Read the model definition and answer for the solid it produces. Units are mm, in the model's axes. Face numbers are marked on the shaded views. A direction names the side the tool comes from. Give positions to 0.01 mm unless a question says otherwise; leave off trailing zeros. Order: outer loops, then holes, each group sorted by start corner. A loop starts at its lowest first (then second) coordinate and runs counter-clockwise, first axis right, second up. Notation, with made-up numbers: (14.25, 9) - (58.25, 9) arc R18 cw to (58.25, 25) - close; hole circle Ø8 at (40, 17.25). An arc over 180 degrees is marked (long way). Answer as CSV lines item,"result". Start each with the question number.
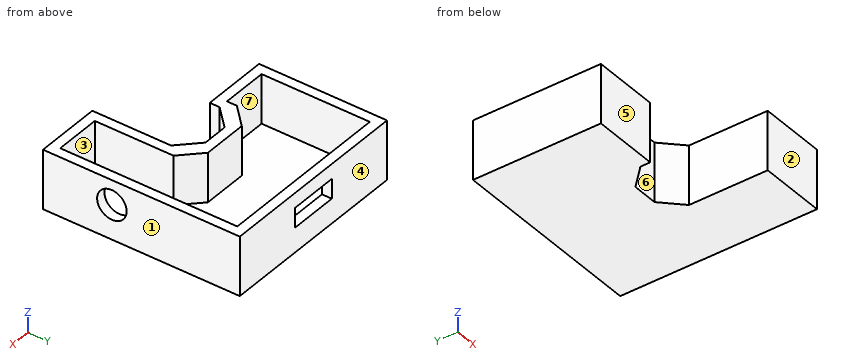
from build123d import *

# Parameters (mm, degrees)
BOSS_EXTRUDE1_DEPTH = 12.5
BOSS_EXTRUDE2_DEPTH = 5
SKETCH3_W           = 25
SKETCH3_H           = 10
CUT_EXTRUDE1_DEPTH  = 109.771549589
SKETCH4_R           = 7.5
CUT_EXTRUDE2_DEPTH  = 10
CHAMFER2_SIZE       = 10
CHAMFER3_SIZE       = 10


with BuildPart() as part:
    # Sketch1 → Boss-Extrude1 (new, symmetric)
    with BuildSketch(Plane.XY):
        Polygon((50, -50), (16.5, -50), (16.5, -45), (16.5, 0), (-16.5, 0), (-16.5, -15), (-50, -15), (-50, 50), (50, 50), align=None)
        Polygon((45, -45), (45, 45), (-45, 45), (-45, -10), (-21.5, -10), (-21.5, 5), (21.5, 5), (21.5, -45), align=None, mode=Mode.SUBTRACT)
    extrude(amount=BOSS_EXTRUDE1_DEPTH, both=True)

    # Sketch2 → Boss-Extrude2 (add)
    with BuildSketch(Plane(origin=(0, 0, -12.5), x_dir=(-1, 0, 0), z_dir=(0, 0, -1))):
        Polygon((-16.5, 0), (16.5, 0), (16.5, -15), (50, -15), (50, 50), (-50, 50), (-50, -50), (-16.5, -50), align=None)
    extrude(amount=BOSS_EXTRUDE2_DEPTH)

    # Sketch3 → Cut-Extrude1 (cut, through all)
    with BuildSketch(Plane.XZ.offset(-45)):
        Rectangle(SKETCH3_W, SKETCH3_H)
    extrude(amount=-CUT_EXTRUDE1_DEPTH, mode=Mode.SUBTRACT)

    # Sketch4 → Cut-Extrude2 (cut)
    with BuildSketch(Plane(origin=(50, 0, 0), x_dir=(0, 0, -1), z_dir=(1, 0, 0))):
        with Locations(Location((0, -15, 0), (0, 0, 90))):
            Circle(SKETCH4_R)
    extrude(amount=-CUT_EXTRUDE2_DEPTH, mode=Mode.SUBTRACT)

    # Chamfer2
    chamfer2_edges = [part.edges().sort_by_distance(p)[0] for p in [
        (16.5, 0, -2.5),
        (-16.5, 0, -2.5),
    ]]
    chamfer(chamfer2_edges, length=CHAMFER2_SIZE)

    # Chamfer3
    chamfer3_edges = [part.edges().sort_by_distance(p)[0] for p in [
        (-21.5, 5, 0),
        (21.5, 5, 0),
    ]]
    chamfer(chamfer3_edges, length=CHAMFER3_SIZE)


solid = part.part
(1) Straight lines are drawn through the part: line 1 (X direction, y = 44, z = 8.5); line 2 (Y direction, x = -39, z = -9); line 3 (X direction, y = -25, z = 2.5). For each, find the intervals that lie inside material, in ascending order. Write a range as [from, to].
(2) Section B-B, the plane y = -36 is taken. Write down the section's boundary in (x, z), and give its area (4 significant figures).
(3) Section D-D, the plane z = -11 is taken. Write down the section's boundary in (x, y), and give its area (3 significant figures).
(4) Determine the mould class of the marked faces 1, 2 and 3 for opening direction X: released by +X, released by -X, zero draft, split by the parting line, or undercut.
(5) Flat-ended cylindrical pins translate along their axes: pin 1 Ø1 at (x, y) = (11, 27.5) entering from +Z; pin 2 Ø10.5 at (x, z) = (-2.5, -0.5) entering from -Y; pin 3 Ø2.5 at (y, z) = (-13.5, 2.5) entering from +X. Find the tip coordinate at first contact, or state that the pin passes through.
(6) Which of the six approach directions +Z, -Z, +X, -X, +Y, -Y give full straight-line access (tool end or side, diameter ignored) to the marked faces 4, 5, 6 and 7?
(7) Section A-A, the plane z = 0 is taken. Write down the section's boundary in (x, y).
(8) Section C-C, the plane x = -32.5 is taken. Write down the section's boundary in (y, z).
Checks:
1,line 1,"x = [-50, -45], [45, 50]"
1,line 2,"y = [-15, -10], [45, 50]"
1,line 3,"x = [16.5, 21.5], [45, 50]"
2,outline,"(16.5, -17.5) - (50, -17.5) - (50, 12.5) - (45, 12.5) - (45, -12.5) - (21.5, -12.5) - (21.5, 12.5) - (16.5, 12.5) - close"
2,area,"417.5 mm²"
3,outline,"(-50, -15) - (-16.5, -15) - (-16.5, -10) - (-6.5, 0) - (6.5, 0) - (16.5, -10) - (16.5, -50) - (50, -50) - (50, 50) - (-50, 50) - close; hole (-45, -10) - (-21.5, -10) - (-21.5, -5) - (-11.5, 5) - (11.5, 5) - (21.5, -5) - (21.5, -45) - (45, -45) - (45, 45) - (-45, 45) - close"
3,area,"2,050 mm²"
4,face 1,"released by +X"
4,face 2,"zero draft"
4,face 3,"undercut"
5,pin 1,"stops at z = -12.5"
5,pin 2,"stops at y = -1.25"
5,pin 3,"stops at x = 21.5"
6,face 4,"+Z, -Z, +X, -X, +Y"
6,face 5,"+Z, -Z, -X, -Y"
6,face 6,"+Z, -Z, -Y"
6,face 7,"+Z"
7,outline,"(-50, -15) - (-16.5, -15) - (-16.5, -10) - (-6.5, 0) - (6.5, 0) - (16.5, -10) - (16.5, -50) - (50, -50) - (50, -22.5) - (45, -22.5) - (45, -45) - (21.5, -45) - (21.5, -5) - (11.5, 5) - (-11.5, 5) - (-21.5, -5) - (-21.5, -10) - (-45, -10) - (-45, 45) - (-12.5, 45) - (-12.5, 50) - (-50, 50) - close; (12.5, 45) - (45, 45) - (45, -7.5) - (50, -7.5) - (50, 50) - (12.5, 50) - close"
8,outline,"(-15, -17.5) - (50, -17.5) - (50, 12.5) - (45, 12.5) - (45, -12.5) - (-10, -12.5) - (-10, 12.5) - (-15, 12.5) - close"
